```python
from build123d import *

# Parameters (mm, degrees)
CROQUIS1_W              = 36
CROQUIS1_H              = 45
SALIENTE_EXTRUIR1_DEPTH = 2
CROQUIS2_W              = 2
CROQUIS2_H              = 11
CROQUIS2_H_2            = 11.033856499
SALIENTE_EXTRUIR2_DEPTH = 18
CROQUIS3_R              = 2.5
CORTAR_EXTRUIR1_DEPTH   = 33


with BuildPart() as part:
    # Croquis1 → Saliente-Extruir1 (new body)
    with BuildSketch(Plane(origin=(0, 0, 0), x_dir=(1, 0, 0), z_dir=(0, 1, 0))):
        Rectangle(CROQUIS1_W, CROQUIS1_H)
    extrude(amount=SALIENTE_EXTRUIR1_DEPTH)

    # Croquis2 → Saliente-Extruir2 (add)
    with BuildSketch(Plane(origin=(0, 2, 0), x_dir=(1, 0, 0), z_dir=(0, 1, 0))):
        with Locations((11.7, -0.033856499)):
            Rectangle(CROQUIS2_W, CROQUIS2_H)
        with Locations((-16, -0.01692825)):
            Rectangle(CROQUIS2_W, CROQUIS2_H_2)
    extrude(amount=-SALIENTE_EXTRUIR2_DEPTH)

    # Croquis3 → Cortar-Extruir1 (cut)
    with BuildSketch(Plane(origin=(12.7, 0, 0), x_dir=(0, 0, -1), z_dir=(1, 0, 0))):
        with Locations((-0.033856499, -10.94)):
            Circle(CROQUIS3_R)
    extrude(amount=-CORTAR_EXTRUIR1_DEPTH, mode=Mode.SUBTRACT)


solid = part.part
```
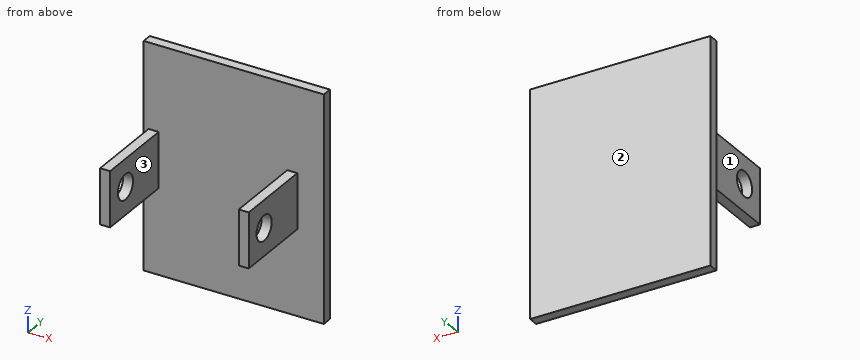
Geometry: final body of the model. Coordinates: model frame, mm. Face numbers are marked on the shaded views. Round coordinates to 2 decimals unless told otherwise and drop trailing zeros. Loops run counter-clockwise (first coordinate to the right, second up) from the corner with the lowest first, then second, coordinate; pieces in that order, holes last. Notation, with made-up numbers: (58.5, 0) -> (91.5, 0) arc R25 cw to (91.5, 29) -> close; hole circle Ø10 at (48, 61.25). An arc over 180 degrees is marked (long way). Use one line per item in the form item = value. Start each with the question number.
1) Section A-A on y = -10.94. Output: boundary loops of the cut face in (x, z), then the cut area to 3 significant figures.
2) Section D-D on x = 13.5. Output: boundary loops of the cut face in (y, z).
3) Line query: L1, parallel to X at y = -8.5, z = -4.5; L2, parallel to Y at x = 6, z = 10.5; L3, parallel to Z at x = 12, y = -7.75. Output: solid intervals per line, ascending.
4) Draft query along X for the marked faces 1, 2 and 3. Return one class per face: released by +X, released by -X, zero draft, split by the parting line, or undercut.
5) Section B-B on z = 0.5. Output: boundary loops of the cut face in (x, y), then the cut area to 3 significant figures.
6) Section C-C on y = -7.5. Output: boundary loops of the cut face in (x, z), then the cut area to 3 significant figures.
7) First-contact query: P1, Ø1.5, axis at x = -7.5, z = 12, coming from the -Y side; P2, Ø2, axis at x = -15.5, y = -9, coming from the -Z side; P3, Ø3.5, axis at y = -9.5, z = -2.5, coming from the +X side; P4, Ø3, axis at y = -10.94, z = 0.03, coming from the -X side. Flat tips, straight axial feed; report the tip coordinate or a pass-through.
Response:
q1.outline = (-17, -5.5) -> (-15, -5.5) -> (-15, -2.47) -> (-17, -2.47) -> close; (-17, 2.53) -> (-15, 2.53) -> (-15, 5.53) -> (-17, 5.53) -> close; (10.7, -5.47) -> (12.7, -5.47) -> (12.7, -2.47) -> (10.7, -2.47) -> close; (10.7, 2.53) -> (12.7, 2.53) -> (12.7, 5.53) -> (10.7, 5.53) -> close
q1.area = 24.1 mm^2
q2.outline = (0, -22.5) -> (2, -22.5) -> (2, 22.5) -> (0, 22.5) -> close
q3.L1 = -17 to -15, 10.7 to 12.7
q3.L2 = 0 to 2
q3.L3 = -5.47 to 5.53
q4.face_1 = released by -X
q4.face_2 = zero draft
q4.face_3 = undercut
q5.outline = (-18, 0) -> (-17, 0) -> (-17, -8.48) -> (-15, -8.48) -> (-15, 0) -> (10.7, 0) -> (10.7, -8.48) -> (12.7, -8.48) -> (12.7, 0) -> (18, 0) -> (18, 2) -> (-18, 2) -> close; (-17, -16) -> (-15, -16) -> (-15, -13.4) -> (-17, -13.4) -> close; (10.7, -16) -> (12.7, -16) -> (12.7, -13.4) -> (10.7, -13.4) -> close
q5.area = 116 mm^2
q6.outline = (-17, -5.5) -> (-15, -5.5) -> (-15, 5.53) -> (-17, 5.53) -> close; (10.7, -5.47) -> (12.7, -5.47) -> (12.7, 5.53) -> (10.7, 5.53) -> close
q6.area = 44.1 mm^2
q7.P1 = 0
q7.P2 = -5.5
q7.P3 = 12.7
q7.P4 = through
